Design review of the part built by this model. Coordinates are the model's own, in mm. Round coordinates to 2 decimals unless told otherwise and drop trailing zeros. Order: outer loops, then holes, each group sorted by start corner. A loop starts at its lowest first (then second) coordinate and runs counter-clockwise, first axis right, second up. Notation, with made-up numbers: M -35.5,79.5 L -30.5,79.5 A9 cw -30.5,84.5 Z; hole C -35.5,2.5 d6. An arc over 180 degrees is marked long. Write each question's results on one line, items separated by ' | '. Start each with the question number.
Item 1: Take a section at A-A, the plane z = -16.5. Write out the cut boundary in (x, y), plus the area to 3 significant figures.
Item 2: Take a section at C-C, the plane y = 6.5. Count the separate pieces of the cut face and the enclosed holes in it, plus the area to 3 significant figures.
Item 3: Clearance check with flat-ended pins moving along their axes: pin 1 (5 mm diameter, centred on x = -40.5, z = 12, fed in from -Y); pin 2 (8 mm diameter, centred on x = 126, z = 21, fed in from -Y). State where each tip first meets the part, or that it passes through.
Item 4: Take a section at D-D, the plane x = 7.5. Write out the cut boundary in (y, z).
Item 5: Wall thickness on line 1 (X direction, y = 2.5, z = 29); line 2 (X direction, y = 5.5, z = 1.5); line 3 (Z direction, x = 86.5, y = 3.25): over which ranges is each line inside the solid? List them lowest first. Write a range as [from, to].
Item 6: Take a section at B-B, the plane x = 155. Write out the cut boundary in (y, z), plus the area to 3 significant figures.
```python
from build123d import *

# Parameters (mm, degrees)
SKETCH_1_W          = 460
SKETCH_1_H          = 90
EXTRUDE_1_DEPTH     = 8
SKETCH_3_W          = 24
SKETCH_3_H          = 30
CUT_EXTRUDE_2_DEPTH = 235.49733474
SKETCH_2_W          = 24
SKETCH_2_H          = 35
CUT_EXTRUDE_3_DEPTH = 235.49733474
FILLET_1_R          = 10
SKETCH_19_R         = 2.5
CUT_EXTRUDE_4_DEPTH = 235.49733474
SKETCH_20_R         = 1.5
CUT_EXTRUDE_5_DEPTH = 235.49733474


with BuildPart() as part:
    # 草图1 → 凸台-拉伸1 (new body)
    with BuildSketch(Plane(origin=(0, 0, 0), x_dir=(1, 0, 0), z_dir=(0, 1, 0))):
        Rectangle(SKETCH_1_W, SKETCH_1_H)
    extrude(amount=EXTRUDE_1_DEPTH)

    # 草图3 → 切除-拉伸2 (cut, through all)
    with BuildSketch(Plane(origin=(0, 8, 0), x_dir=(1, 0, 0), z_dir=(0, 1, 0))):
        with Locations((120, -30)):
            Rectangle(SKETCH_3_W, SKETCH_3_H)
        Polygon((-70, 45), (70, 45), (48.5526258, 25), (-48.5526258, 25), align=None)
    cut_extrude_2 = extrude(amount=-CUT_EXTRUDE_2_DEPTH, mode=Mode.SUBTRACT)

    # 草图2 → 切除-拉伸3 (cut, through all)
    with BuildSketch(Plane(origin=(0, 8, 0), x_dir=(1, 0, 0), z_dir=(0, 1, 0))):
        with Locations((152, 17.5)):
            Rectangle(SKETCH_2_W, SKETCH_2_H)
        with Locations((96, 17.5)):
            Rectangle(SKETCH_2_W, SKETCH_2_H)
    cut_extrude_3 = extrude(amount=-CUT_EXTRUDE_3_DEPTH, mode=Mode.SUBTRACT)

    # 镜向1: 切除-拉伸2, 切除-拉伸3 across plane
    add(cut_extrude_2.mirror(Plane(origin=(0, 0, 0), x_dir=(0, 0, 1), z_dir=(1, 0, 0))), mode=Mode.SUBTRACT)
    add(cut_extrude_3.mirror(Plane(origin=(0, 0, 0), x_dir=(0, 0, 1), z_dir=(1, 0, 0))), mode=Mode.SUBTRACT)

    # 圆角1
    fillet_1_edges = [part.edges().sort_by_distance(p)[0] for p in [
        (-48.5526258, 4, -25),
        (-70, 4, -45),
        (70, 4, -45),
        (48.5526258, 4, -25),
        (-230, 4, -45),
        (230, 4, -45),
    ]]
    fillet(fillet_1_edges, radius=FILLET_1_R)

    # 草图19 → 切除-拉伸4 (cut, through all)
    with BuildSketch(Plane(origin=(0, 8, 0), x_dir=(1, 0, 0), z_dir=(0, 1, 0))):
        with Locations(Location((-120, 5, 0), (0, 0, 270))):
            Circle(SKETCH_19_R)
        with Locations(Location((-120, 25, 0), (0, 0, 270))):
            Circle(SKETCH_19_R)
    cut_extrude_4 = extrude(amount=-CUT_EXTRUDE_4_DEPTH, mode=Mode.SUBTRACT)

    # 镜向2: 切除-拉伸4 across plane
    add(cut_extrude_4.mirror(Plane(origin=(0, 0, 0), x_dir=(0, 0, 1), z_dir=(1, 0, 0))), mode=Mode.SUBTRACT)

    # 草图20 → 切除-拉伸5 (cut, through all)
    with BuildSketch(Plane(origin=(0, 8, 0), x_dir=(1, 0, 0), z_dir=(0, 1, 0))):
        with Locations(Location((-215, 30, 0), (0, 0, 270))):
            Circle(SKETCH_20_R)
        with Locations(Location((-215, -1.5, 0), (0, 0, 270))):
            Circle(SKETCH_20_R)
        with Locations(Location((-215, -33, 0), (0, 0, 270))):
            Circle(SKETCH_20_R)
        with Locations(Location((-70, 25, 0), (0, 0, 270))):
            Circle(SKETCH_20_R)
        with Locations(Location((-70, -33, 0), (0, 0, 270))):
            Circle(SKETCH_20_R)
        with Locations(Location((-170, -33, 0), (0, 0, 270))):
            Circle(SKETCH_20_R)
    cut_extrude_5 = extrude(amount=-CUT_EXTRUDE_5_DEPTH, mode=Mode.SUBTRACT)

    # 镜向3: 切除-拉伸5 across plane
    add(cut_extrude_5.mirror(Plane(origin=(0, 0, 0), x_dir=(0, 0, 1), z_dir=(1, 0, 0))), mode=Mode.SUBTRACT)


solid = part.part
```
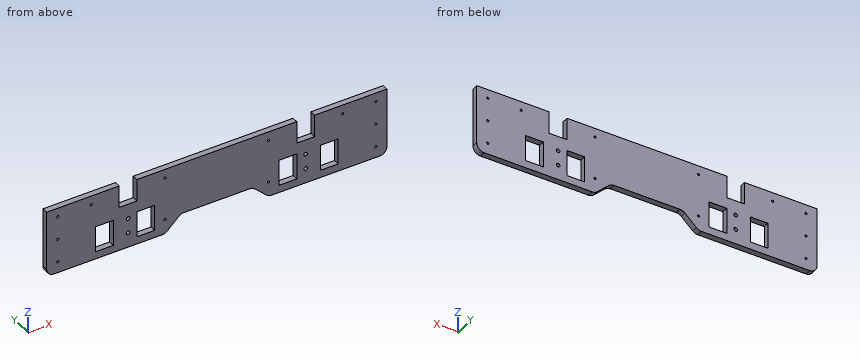
Results list:
1) outline: M -230,0 L -164,0 L -164,8 L -230,8 Z; M -140,0 L -108,0 L -108,8 L -140,8 Z; M -84,0 L 84,0 L 84,8 L -84,8 Z; M 108,0 L 140,0 L 140,8 L 108,8 Z; M 164,0 L 230,0 L 230,8 L 164,8 Z | area: 2,910 mm²
2) separate pieces: 1 | enclosed holes: 20 | area: 34,000 mm²
3) pin 1: y = 0 | pin 2: through
4) outline: M 0,-25 L 8,-25 L 8,45 L 0,45 Z
5) line 1: [-230, -132], [-108, 108], [132, 230] | line 2: [-230, -216.5], [-213.5, 213.5], [216.5, 230] | line 3: [-45, -35], [0, 45]
6) outline: M 0,-45 L 8,-45 L 8,-35 L 0,-35 Z; M 0,0 L 8,0 L 8,45 L 0,45 Z | area: 440 mm²
